Autodesk Inventor part; units mm, degrees
ref_plane "Work Plane2" through (-18, -2, 8) normal (0, 0, -1) x (0, 1, 0)
ref_plane "Work Plane3" through (-18, -2, 8) normal (0, 0, -1) x (0, 1, 0)
ref_plane "Work Plane5" through (-45.5, 1, 28.397) normal (0, -1, 0) x (1, 0, 0)
ref_plane "Work Plane1" through (0, 0, 0) normal (0, 0, 1) x (1, 0, 0)
sketch "Sketch1" plane through (0, 0, 0) normal (0, 0, 1) x (1, 0, 0)
  circle A0 centre (0, 25) radius 1.95 construction
  circle A1 centre (-25, 0) radius 1.95 construction
  circle A2 centre (-25, -25) radius 1.95 construction
  circle A3 centre (25, 25) radius 1.95 construction
  circle A4 centre (25, -25) radius 1.95 construction
  circle A5 centre (-25, 25) radius 1.95 construction
  circle A6 centre (25, 0) radius 1.95 construction
  circle A7 centre (0, -25) radius 1.95 construction
  line L0 (-28, 30) -> (-30, 28)
  line L1 (-30, 28) -> (-30, -28)
  line L2 (-30, -28) -> (-28, -30)
  line L3 (-28, -30) -> (28, -30)
  line L4 (28, -30) -> (30, -28)
  line L5 (30, -28) -> (30, 28)
  line L6 (30, 28) -> (28, 30)
  line L7 (28, 30) -> (-28, 30)
  circle A8 centre (25, 25) radius 1.45
  circle A9 centre (25, -25) radius 1.45
  circle A10 centre (-25, -25) radius 1.45
  circle A11 centre (-25, 25) radius 1.45
  circle A12 centre (0, 25) radius 1.95
  circle A13 centre (-25, 0) radius 1.95
  circle A14 centre (-25, -25) radius 1.95
  circle A15 centre (25, 25) radius 1.95
  circle A16 centre (25, -25) radius 1.95
  circle A17 centre (-25, 25) radius 1.95
  circle A18 centre (25, 0) radius 1.95
  circle A19 centre (0, -25) radius 1.95
  line L8 (-28, 30) -> (-30, 28)
  line L9 (-30, 28) -> (-30, -28)
  line L10 (-30, -28) -> (-28, -30)
  line L11 (-28, -30) -> (28, -30)
  line L12 (28, -30) -> (30, -28)
  line L13 (30, -28) -> (30, 28)
  line L14 (30, 28) -> (28, 30)
  line L15 (28, 30) -> (-28, 30)
  line L16 (-44.5, 28.8555) -> (-44.5, 2)
  line L17 (-44.5, 34) -> (-45.5, 34)
  line L18 (-45.5, 1) -> (-44.5, 1)
  line L19 (-44.5, 34) -> (-30, 34)
  line L20 (-30, 34) -> (-30, 1)
  line L21 (-30, 1) -> (-44.5, 1)
  line L22 (-44.5, 1) -> (-44.5, 34)
  line L23 (-30, 34) -> (-26, 30)
  line L24 (-30, 34) -> (-24.3431, 34) construction
  point P0 (0, 0)
  dimension "d0" = 2.9
  dimension "d1" = 2.9
  dimension "d2" = 2.9
  dimension "d3" = 2.9
  dimension "d6" = 45
ref_plane "Work Plane2" through (-18, -2, 8) normal (0, 0, -1) x (0, 1, 0)
extrude "Extrusion1" add sketch "Sketch1" along normal blind 3 contours L7 L6 L5 L4 L3 L2 L1 L0 | A12 | A13 | A14 | A15 | A16 | A17 | A18 | A19
sketch "Sketch2" plane through (0, 0, 3) normal (0, 0, 1) x (1, 0, 0)
  circle A0 centre (-3, 22) radius 1.4
  circle A1 centre (-3, 14) radius 1.4
  circle A2 centre (-13, 6) radius 1.4
  circle A3 centre (-13, 14) radius 1.4
  circle A4 centre (25, 14) radius 1.4
  circle A5 centre (25, 6) radius 1.4
  circle A6 centre (-13, 22) radius 1.4
  circle A7 centre (-3, 6) radius 1.4
  circle A8 centre (25, 22) radius 1.4
  line L0 (30, -2) -> (30, 30)
  line L1 (30, -2) -> (-18, -2)
  line L2 (-18, 30) -> (-18, -2)
  line L3 (30, 30) -> (-18, 30)
  point P0 (0, 0)
ref_plane "Work Plane3" through (-18, -2, 8) normal (0, 0, -1) x (0, 1, 0)
extrude "Extrusion2" add sketch "Sketch2" along normal up to surface (5 mm away)
sketch "Sketch3" plane through (0, 0, 0) normal (0, 0, -1) x (-1, 0, 0)
  circle A0 centre (-25, 22) radius 1.4
  circle A1 centre (3, 6) radius 1.4
  circle A2 centre (13, 22) radius 1.4
  circle A3 centre (-25, 6) radius 1.4
  circle A4 centre (-25, 14) radius 1.4
  circle A5 centre (13, 14) radius 1.4
  circle A6 centre (13, 6) radius 1.4
  circle A7 centre (3, 14) radius 1.4
  circle A8 centre (3, 22) radius 1.4
  line L0 (18, -2) -> (-30, -2)
  line L1 (-30, -2) -> (-30, 30)
  line L2 (-30, 30) -> (18, 30)
  line L3 (18, 30) -> (18, -2)
  point P0 (0, 0)
hole "Hole2" at (-13, 6, 0) at (-13, 14, 0) at (-13, 22, 0) at (-3, 22, 0) at (-3, 14, 0) at (-3, 6, 0) at (25, 6, 0) at (25, 14, 0) at (25, 22, 0) direction (0, 0, 1) diameter 3.2 depth 20 tip angle 118 counterbore diameter 5 counterbore depth 4
ref_plane "Work Plane4" through (-44.5, 34, 36.7) normal (0, 1, 0) x (0, 0, -1)
sketch "Sketch5" plane through (-44.5, 34, 36.7) normal (0, 1, 0) x (0, 0, -1)
  line L0 (36.7, -72.5) -> (36.7, -16.5)
  line L1 (36.7, -16.5) -> (33.7, -16.5)
  line L2 (33.7, -26.5) -> (33.7, -16.5)
  line L3 (33.7, -26.5) -> (28.7, -26.5)
  line L4 (28.7, -74.5) -> (28.7, -26.5)
  line L5 (33.7, -74.5) -> (28.7, -74.5)
  line L6 (33.7, -74.5) -> (33.7, -72.5)
  line L7 (36.7, -72.5) -> (33.7, -72.5)
  line L8 (25.7, 0) -> (0, 0)
  line L9 (25.7, 0) -> (25.7, 1)
  line L10 (0, 1) -> (25.7, 1)
  line L11 (0, 0) -> (0, 1)
  line L12 (0, 0) -> (24, 0)
  line L13 (24, 0) -> (24, -4)
  line L14 (24, -4) -> (0, -4)
  line L15 (0, -4) -> (0, 0)
  line L16 (24, -4) -> (33.7, -16.5)
  line L17 (36.7, -16.5) -> (36.7, -14.5)
  line L18 (36.7, -14.5) -> (36.7, -16.5)
  line L19 (24, 0) -> (36.7, -14.5)
  line L20 (36.7, -16.5) -> (33.7, -16.5)
  line L21 (36.7, -14.5) -> (36.7, -16.5)
  point P0 (36.7, -44.5)
  dimension "d23" = 24
  dimension "d24" = 4
ref_plane "Work Plane5" through (-45.5, 1, 28.397) normal (0, -1, 0) x (1, 0, 0)
extrude "Extrusion3" add sketch "Sketch5" against normal up to surface (33 mm away) contours L1 L16 L13 L19 L17 | L14 L15 L8 L13
sketch "Sketch6" plane through (-44.5, 34, 36.7) normal (0, 1, 0) x (1, 0, 0)
  line L0 (0, 0) -> (0, 24)
  line L1 (4, 0) -> (0, 0)
  line L2 (4, 24) -> (4, 0)
  line L3 (16.5, 33.7) -> (4, 24)
  line L4 (26.5, 33.7) -> (26.5, 28.7)
  line L5 (26.5, 28.7) -> (4, 0)
  line L6 (0, 24) -> (14.5, 36.7)
  line L7 (14.5, 36.7) -> (16.5, 36.7)
  line L8 (16.5, 36.7) -> (16.5, 33.7)
  line L9 (26.5, 33.7) -> (26.5, 28.7)
  line L10 (16.5, 36.7) -> (26.5, 36.7)
  line L11 (26.5, 36.7) -> (26.5, 28.7)
  line L12 (26.5, 28.7) -> (16.5, 28.7)
  line L13 (16.5, 28.7) -> (16.5, 36.7)
  point P0 (44.5, 36.7)
extrude "Extrusion4" add sketch "Sketch6" against normal blind 2
sketch "Sketch7" plane through (-44.5, 1, 36.7) normal (-1, 0, 0) x (0, 0, 1)
  circle A0 centre (-7.7, 2.5) radius 1
  circle A1 centre (-2.7, 30.5) radius 1
  circle A2 centre (-23.2, 24) radius 1
  circle A3 centre (-12.7, 13) radius 2.6486
  line L0 (-18.1576, 5.885) -> (-7.0605, 5.885)
  line L1 (-7.0605, 5.885) -> (-7.0605, 20.8532)
  line L2 (-7.0605, 20.8532) -> (-18.1576, 20.8532)
  line L3 (-18.1576, 20.8532) -> (-18.1576, 5.885)
  point P0 (-36.7, -1)
extrude "Extrusion5" cut sketch "Sketch7" against normal through all contours A0 | A1 | A2 | A3 | L3 L2 L1 L0
sketch "Sketch8" plane through (0, 0, 0) normal (0, 0, -1) x (-1, 0, 0)
  line L0 (28, 32) -> (28, 30)
  line L1 (-28, 30) -> (28, 30)
  line L2 (-30, 28) -> (-28, 30)
  line L3 (-30, -28) -> (-30, 28)
  line L4 (-28, -30) -> (-30, -28)
  line L5 (28, -30) -> (-28, -30)
  line L6 (30, -28) -> (28, -30)
  line L7 (30, 1) -> (30, -28)
  line L8 (30, 34) -> (30, 1)
  line L9 (30, 34) -> (18, 34)
  line L10 (18, 34) -> (18, 32)
  line L11 (28, 32) -> (18, 32)
  circle A0 centre (25, -25) radius 1.45
  arc A1 (-26.2035, 24.1913) -> (-23.7965, 24.1913) centre (-25, 22) ccw
  arc A2 (-23.7965, 24.1913) -> (-26.2035, 24.1913) centre (-25, 25) ccw
  circle A3 centre (-25, -25) radius 1.45
  circle A4 centre (25, 25) radius 1.45
  circle A5 centre (-25, 6) radius 2.5
  circle A6 centre (3, 14) radius 2.5
  circle A7 centre (13, 22) radius 2.5
  circle A8 centre (13, 6) radius 2.5
  circle A9 centre (13, 14) radius 2.5
  circle A10 centre (3, 22) radius 2.5
  circle A11 centre (3, 6) radius 2.5
  circle A12 centre (-25, 14) radius 2.5
  line L12 (18, 34) -> (18, 32)
  line L13 (18, 34) -> (14, 30)
  line L14 (18, 34) -> (23.6569, 34) construction
  line L15 (-28, 30) -> (28, 30)
  point P0 (0, 0)
  dimension "d31" = 135
extrude "Extrusion6" add sketch "Sketch8" against normal up to surface (8 mm away) contours L0 L1 L13 L10 L11
properties part number "cellSTORM_inverted_Laser_left"
Verification items for the finished model (mm, model axes). A direction names the side the tool comes from. Give positions to 0.01 mm unless a question says otherwise; leave off trailing zeros. Loops run counter-clockwise (first coordinate to the right, second up) from the corner with the lowest first, then second, coordinate; pieces in that order, holes last.
1) Depth check by flat-ended pin: pin 1 Ø18 at (x, z) = (-34.5, 14) entering from -Y; pin 2 Ø11 at (x, y) = (-8.5, 22.5) entering from +Z; pin 3 Ø12 at (x, y) = (-0.5, -18) entering from +Z; pin 4 Ø3 at (x, y) = (-13, 6) entering from +Z. Enter the tip coordinate at first touch or a pass-through.
2) Thickness scan on line 1 along Y through (x, z) = (-3, 5); line 2 along Y through (x, z) = (25, 1); line 3 along Y through (x, z) = (-3, 1). Record the ranges inside material, lowest first.
3) Sectioned sample at A-A, the plane y = 6. Count the separate pieces of the cut face and the enclosed holes in it, then the cut area to 3 significant figures.
4) Draft check along Y on faces 6 (the flat face through (1, 16, 8)), 7 (the flat face through (0, -30, 1)), 8 (the cylindrical face through (24.96, 26.45, 1.48)), 9 (the flat face through (-16, 32, 4)). Enter one of: pulls with the +Y half, pulls with the -Y half, needs draft (parallel to the pull), parting line crosses it, or undercut.
5) Sectioned sample at C-C, the plane z = 27. Enter the section's corners in (x, y) (3 decimals), then the cut area to 3 significant figures.
6) Set-up check for faces 1 (the flat face through (-42, 18, 36.7)), 2 (the flat face through (-34.34, 16.72, 7.92)), 3 (the flat face through (0, 2, 0)), 4 (the cylindrical face through (-3.1, 19.5, 2)), 5 (the flat face through (-30, -13, 1)): record each of +Z, -Z, +X, -X, +Y, -Y from which the full face is reachable in a straight line by a thin tool's end or side.
Answers:
1. pin 1: stops at y = 1
1. pin 2: stops at z = 8
1. pin 3: stops at z = 3
1. pin 4: passes through
2. line 1: y = -2 to 4.4, 7.6 to 12.4, 15.6 to 20.4, 23.6 to 30
2. line 2: y = -30 to -26.45, -23.55 to 3.5, 8.5 to 11.5, 16.5 to 19.5, 26.45 to 30
2. line 3: y = -30 to 3.5, 8.5 to 11.5, 16.5 to 19.5, 24.5 to 30
3. separate pieces: 4
3. enclosed holes: 0
3. area: 468 mm2
4. face 6: needs draft
4. face 7: pulls with the -Y half
4. face 8: undercut
4. face 9: pulls with the +Y half
5. outline: (-44.5, 1) - (-40.5, 1) - (-40.5, 6.885) - (-44.5, 6.885) - close; (-44.5, 21.853) - (-40.5, 21.853) - (-40.5, 32) - (-32.895, 32) - (-32.895, 34) - (-44.5, 34) - close
5. area: 87.3 mm2
6. face 1: +Z, +X, -X, +Y, -Y
6. face 2: +Z, -Y
6. face 3: -Z, +X, -X, +Y, -Y
6. face 4: -Z
6. face 5: +Z, -Z, -X, -Y
